```python
from build123d import *

# Parameters (mm, degrees)
F1_DEPTH = 6.35
F2_R     = 2.53999


# Not quite as in the source:
# - a fillet or chamfer is up to 0.001 mm smaller than in the source, because OpenCascade refuses the exact size


with BuildPart() as f1:
    # F0 (on Top) → F1 (new body)
    with BuildSketch(Plane.XY):
        with BuildLine():
            ThreePointArc((6.76275, -11.7134265989), (11.7134265989, -6.76275), (13.5255, 0))
            ThreePointArc((13.5255, 0), (11.7134265989, 6.76275), (6.76275, 11.7134265989))
            ThreePointArc((6.76275, 11.7134265989), (3.5006569945, 13.0646297635), (0, 13.5255))
            Line((0, 13.5255), (0, 10.9855))
            ThreePointArc((0, 10.9855), (7.7679215447, 7.7679215447), (10.9855, 0))
            ThreePointArc((10.9855, 0), (7.7679215447, -7.7679215447), (0, -10.9855))
            Line((0, -10.9855), (0, -13.5255))
            ThreePointArc((0, -13.5255), (3.5006569945, -13.0646297635), (6.76275, -11.7134265989))
        make_face()
        with BuildLine():
            Line((13.5255, -7.8089510659), (13.5255, 0))
            ThreePointArc((13.5255, 0), (11.7134265989, -6.76275), (6.76275, -11.7134265989))
            Line((6.76275, -11.7134265989), (13.5255, -7.8089510659))
        make_face()
        with BuildLine():
            ThreePointArc((6.76275, 11.7134265989), (11.7134265989, 6.76275), (13.5255, 0))
            Line((13.5255, 0), (13.5255, 7.8089510659))
            Line((13.5255, 7.8089510659), (6.76275, 11.7134265989))
        make_face()
        with BuildLine():
            ThreePointArc((0, 13.5255), (3.5006569945, 13.0646297635), (6.76275, 11.7134265989))
            Line((6.76275, 11.7134265989), (0.6545456927, 15.24))
            Line((0.6545456927, 15.24), (0, 14.8620978682))
            Line((0, 14.8620978682), (0, 13.5255))
        make_face()
        Polygon((0.6545456927, 15.24), (6.76275, 11.7134265989), (6.76275, 18.7665734011), align=None)
        with BuildLine():
            Line((0.6545456927, -15.24), (6.76275, -11.7134265989))
            ThreePointArc((6.76275, -11.7134265989), (3.5006569945, -13.0646297635), (0, -13.5255))
            Line((0, -13.5255), (0, -14.8620978682))
            Line((0, -14.8620978682), (0.6545456927, -15.24))
        make_face()
        Polygon((6.76275, -18.7665734011), (6.76275, -11.7134265989), (0.6545456927, -15.24), align=None)
        with BuildLine():
            Line((0, 10.9855), (0, 13.5255))
            ThreePointArc((0, 13.5255), (-3.5006569945, 13.0646297635), (-6.76275, 11.7134265989))
            ThreePointArc((-6.76275, 11.7134265989), (-11.7134265989, 6.76275), (-13.5255, 0))
            ThreePointArc((-13.5255, 0), (-11.7134265989, -6.76275), (-6.76275, -11.7134265989))
            ThreePointArc((-6.76275, -11.7134265989), (-3.5006569945, -13.0646297635), (0, -13.5255))
            Line((0, -13.5255), (0, -10.9855))
            ThreePointArc((0, -10.9855), (-10.9855, 0), (0, 10.9855))
        make_face()
        with BuildLine():
            ThreePointArc((-6.76275, 11.7134265989), (-3.5006569945, 13.0646297635), (0, 13.5255))
            Line((0, 13.5255), (0, 14.8620978682))
            Line((0, 14.8620978682), (-0.6545456927, 15.24))
            Line((-0.6545456927, 15.24), (-6.76275, 11.7134265989))
        make_face()
        with BuildLine():
            Line((0, 15.6179021318), (0.6545456927, 15.24))
            Line((0.6545456927, 15.24), (6.76275, 18.7665734011))
            ThreePointArc((6.76275, 18.7665734011), (3.5006569945, 17.4153702365), (0, 16.9545))
            Line((0, 16.9545), (0, 15.6179021318))
        make_face()
        with BuildLine():
            ThreePointArc((0, 16.9545), (3.5006569945, 17.4153702365), (6.76275, 18.7665734011))
            ThreePointArc((6.76275, 18.7665734011), (11.7134265989, 23.71725), (13.5255, 30.48))
            ThreePointArc((13.5255, 30.48), (11.7134266013, 37.2427499958), (6.7627500083, 42.1934265941))
            ThreePointArc((6.7627500083, 42.1934265941), (-1.056e-07, 44.0055), (-6.7627501912, 42.1934264885))
            ThreePointArc((-6.7627501912, 42.1934264885), (-11.7134266541, 37.2427499044), (-13.5255, 30.48))
            ThreePointArc((-13.5255, 30.48), (-11.7134265989, 23.71725), (-6.76275, 18.7665734011))
            ThreePointArc((-6.76275, 18.7665734011), (-3.5006569945, 17.4153702365), (0, 16.9545))
        make_face()
        with BuildLine():
            ThreePointArc((10.9855, 30.48), (7.7679215447, 22.7120784553), (0, 19.4945))
            ThreePointArc((0, 19.4945), (-7.7679215447, 38.2479215447), (10.9855, 30.48))
        make_face(mode=Mode.SUBTRACT)
        with BuildLine():
            ThreePointArc((13.5255, 30.48), (11.7134265989, 23.71725), (6.76275, 18.7665734011))
            Line((6.76275, 18.7665734011), (13.5255, 22.6710489341))
            Line((13.5255, 22.6710489341), (13.5255, 30.48))
        make_face()
        with BuildLine():
            Line((0, -14.8620978682), (0, -13.5255))
            ThreePointArc((0, -13.5255), (-3.5006569945, -13.0646297635), (-6.76275, -11.7134265989))
            Line((-6.76275, -11.7134265989), (-0.6545456927, -15.24))
            Line((-0.6545456927, -15.24), (0, -14.8620978682))
        make_face()
        with BuildLine():
            Line((6.76275, -18.7665734011), (0.6545456927, -15.24))
            Line((0.6545456927, -15.24), (0, -15.6179021318))
            Line((0, -15.6179021318), (0, -16.9545))
            ThreePointArc((0, -16.9545), (3.5006569945, -17.4153702365), (6.76275, -18.7665734011))
        make_face()
        with BuildLine():
            Line((13.5255, -22.6710489341), (6.76275, -18.7665734011))
            ThreePointArc((6.76275, -18.7665734011), (11.7134265989, -23.71725), (13.5255, -30.48))
            Line((13.5255, -30.48), (13.5255, -22.6710489341))
        make_face()
        with BuildLine():
            ThreePointArc((13.5255, -30.48), (11.7134265989, -23.71725), (6.76275, -18.7665734011))
            ThreePointArc((6.76275, -18.7665734011), (3.5006569945, -17.4153702365), (0, -16.9545))
            ThreePointArc((0, -16.9545), (-3.5006569945, -17.4153702365), (-6.76275, -18.7665734011))
            ThreePointArc((-6.76275, -18.7665734011), (-11.7134265989, -23.71725), (-13.5255, -30.48))
            ThreePointArc((-13.5255, -30.48), (-11.7134266419, -37.2427499255), (-6.762750149, -42.1934265129))
            ThreePointArc((-6.762750149, -42.1934265129), (-1.97e-07, -44.0055), (6.7627498078, -42.1934267099))
            ThreePointArc((6.7627498078, -42.1934267099), (11.7134265434, -37.2427500961), (13.5255, -30.48))
        make_face()
        with BuildLine():
            ThreePointArc((10.9855, -30.48), (-7.7679215447, -38.2479215447), (0, -19.4945))
            ThreePointArc((0, -19.4945), (7.7679215447, -22.7120784553), (10.9855, -30.48))
        make_face(mode=Mode.SUBTRACT)
        with BuildLine():
            ThreePointArc((-13.5255, 0), (-11.7134265989, 6.76275), (-6.76275, 11.7134265989))
            Line((-6.76275, 11.7134265989), (-13.5255, 7.8089510659))
            Line((-13.5255, 7.8089510659), (-13.5255, 0))
        make_face()
        Polygon((-6.76275, 18.7665734011), (-6.76275, 11.7134265989), (-0.6545456927, 15.24), align=None)
        with BuildLine():
            Line((-0.6545456927, 15.24), (0, 15.6179021318))
            Line((0, 15.6179021318), (0, 16.9545))
            ThreePointArc((0, 16.9545), (-3.5006569945, 17.4153702365), (-6.76275, 18.7665734011))
            Line((-6.76275, 18.7665734011), (-0.6545456927, 15.24))
        make_face()
        with BuildLine():
            ThreePointArc((6.7627500083, 42.1934265941), (11.7134266013, 37.2427499958), (13.5255, 30.48))
            Line((13.5255, 30.48), (13.5255, 38.2889510659))
            Line((13.5255, 38.2889510659), (6.7627500083, 42.1934265941))
        make_face()
        with BuildLine():
            Line((-13.5255, -7.8089510659), (-6.76275, -11.7134265989))
            ThreePointArc((-6.76275, -11.7134265989), (-11.7134265989, -6.76275), (-13.5255, 0))
            Line((-13.5255, 0), (-13.5255, -7.8089510659))
        make_face()
        Polygon((-0.6545456927, -15.24), (-6.76275, -11.7134265989), (-6.76275, -18.7665734011), align=None)
        with BuildLine():
            Line((0, -16.9545), (0, -15.6179021318))
            Line((0, -15.6179021318), (-0.6545456927, -15.24))
            Line((-0.6545456927, -15.24), (-6.76275, -18.7665734011))
            ThreePointArc((-6.76275, -18.7665734011), (-3.5006569945, -17.4153702365), (0, -16.9545))
        make_face()
        with BuildLine():
            Line((13.5255, -38.2889510659), (13.5255, -30.48))
            ThreePointArc((13.5255, -30.48), (11.7134265434, -37.2427500961), (6.7627498078, -42.1934267099))
            Line((6.7627498078, -42.1934267099), (13.5255, -38.2889510659))
        make_face()
        with BuildLine():
            Line((-13.5255, 22.6710489341), (-6.76275, 18.7665734011))
            ThreePointArc((-6.76275, 18.7665734011), (-11.7134265989, 23.71725), (-13.5255, 30.48))
            Line((-13.5255, 30.48), (-13.5255, 22.6710489341))
        make_face()
        with BuildLine():
            ThreePointArc((-6.7627501912, 42.1934264885), (-1.056e-07, 44.0055), (6.7627500083, 42.1934265941))
            Line((6.7627500083, 42.1934265941), (0, 46.0979021318))
            Line((0, 46.0979021318), (-6.7627501912, 42.1934264885))
        make_face()
        with BuildLine():
            ThreePointArc((-13.5255, -30.48), (-11.7134265989, -23.71725), (-6.76275, -18.7665734011))
            Line((-6.76275, -18.7665734011), (-13.5255, -22.6710489341))
            Line((-13.5255, -22.6710489341), (-13.5255, -30.48))
        make_face()
        with BuildLine():
            Line((0, -46.0979021318), (6.7627498078, -42.1934267099))
            ThreePointArc((6.7627498078, -42.1934267099), (-1.97e-07, -44.0055), (-6.762750149, -42.1934265129))
            Line((-6.762750149, -42.1934265129), (0, -46.0979021318))
        make_face()
        with BuildLine():
            Line((-13.5255, 38.2889510659), (-13.5255, 30.48))
            ThreePointArc((-13.5255, 30.48), (-11.7134266541, 37.2427499044), (-6.7627501912, 42.1934264885))
            Line((-6.7627501912, 42.1934264885), (-13.5255, 38.2889510659))
        make_face()
        with BuildLine():
            ThreePointArc((-6.762750149, -42.1934265129), (-11.7134266419, -37.2427499255), (-13.5255, -30.48))
            Line((-13.5255, -30.48), (-13.5255, -38.2889510659))
            Line((-13.5255, -38.2889510659), (-6.762750149, -42.1934265129))
        make_face()
    extrude(amount=F1_DEPTH)

    # F2 (radius 2.54 in the source; OpenCascade refuses exactly that, so slightly less here)
    f2_edges = [f1.edges().sort_by_distance(p)[0] for p in [
        (-6.76275, -42.193427, 6.35),
        (6.76275, -42.193427, 6.35),
        (13.5255, -30.48, 6.35),
        (-13.5255, -30.48, 6.35),
        (-10.144125, -20.718811, 6.35),
        (-6.76275, -15.24, 6.35),
        (10.144125, -20.718811, 6.35),
        (6.76275, -15.24, 6.35),
        (-10.144125, -9.761189, 6.35),
        (-13.5255, 0, 6.35),
        (-10.144125, 9.761189, 6.35),
        (-6.76275, 15.24, 6.35),
        (-10.144125, 20.718811, 6.35),
        (-13.5255, 30.48, 6.35),
        (-6.76275, 42.193427, 6.35),
        (6.76275, 42.193427, 6.35),
        (13.5255, 30.48, 6.35),
        (6.76275, 15.24, 6.35),
        (10.144125, 20.718811, 6.35),
        (10.144125, 9.761189, 6.35),
        (10.144125, -9.761189, 6.35),
        (13.5255, 0, 6.35),
        (-13.5255, -30.48, 0),
        (-6.76275, -42.193427, 0),
        (6.76275, -42.193427, 0),
        (13.5255, -30.48, 0),
        (10.144125, -20.718811, 0),
        (6.76275, -15.24, 0),
        (-10.144125, -20.718811, 0),
        (-6.76275, -15.24, 0),
        (-13.5255, 0, 0),
        (-10.144125, 9.761189, 0),
        (-6.76275, 15.24, 0),
        (-13.5255, 30.48, 0),
        (-6.76275, 42.193427, 0),
        (6.76275, 42.193427, 0),
        (13.5255, 30.48, 0),
        (10.144125, 20.718811, 0),
        (6.76275, 15.24, 0),
        (10.144125, 9.761189, 0),
        (10.144125, -9.761189, 0),
        (13.5255, 0, 0),
        (-10.144125, 20.718811, 0),
    ]]
    fillet(f2_edges, radius=F2_R)


solid = f1.part
```
For this review, take the finished solid that the model builds, in its own axes (mm). A direction names the side the tool comes from. Give positions to 0.01 mm unless a question says otherwise; leave off trailing zeros. Write each loop counter-clockwise with the first axis right and the second up, starting at its lowest first coordinate (ties: lowest second). Pieces come first, ordered by that corner, then holes. Notation, with made-up numbers: M -24.75,60.5 L 12.25,60.5 A23 ccw 12.25,92.5 Z; hole C 84.5,28.25 d2. An arc over 180 degrees is marked long. Answer as a JSON object with one key per item and string values. Group by question number.
Item 1: Consider section B-B on y = -27. Write out the cut boundary in (x, z).
Item 2: Consider section A-A on y = 34. Write out the cut boundary in (x, z), plus the area to 3 significant figures.
Item 3: Draft analysis for pull direction Y (two halves, no side actions). For faces 5 (the cylindrical face through (-9.203, -21.012, 0.764)), 6 (the cylindrical face through (-12.8, 30.37, 5.59)), state which applies: +Y half, -Y half, draft (parallel to the pull), parting line (faces both ways), or undercut.
Item 4: For pin 1 Ø6 at (x, y) = (-7.5, -24) entering from -Z; pin 2 Ø1 at (y, z) = (-14.5, 3) entering from -X; pin 3 Ø1.4 at (y, z) = (15, 3) entering from +X, all flat-tipped, find the tip position at first contact; note any pin that passes through.
Item 5: For probe 1 along X at (y, z) = (30.48, 3.5); probe 2 along Y at (x, z) = (-5.75, 3.5); probe 3 along Y at (x, z) = (7.5, 1.5), list the stretches that pass through material, from the lowest coordinate up. Write a range as [from, to].
Item 6: Tool access review of faces 1 (the cylindrical face through (6.038, -15.17, 5.586)), 2 (the cylindrical face through (9.09, 9.53, 0.76)), 3 (the cylindrical face through (-6.038, 15.17, 5.586)), 4 (the cylindrical face through (-6.038, 15.17, 0.764)): name each direction out of +Z, -Z, +X, -X, +Y, -Y from which nothing blocks a thin tool from reaching the whole face with its end or side.
Item 7: Consider section C-C on z = 5. Count the separate pieces of the cut face and the enclosed holes in it, plus the area to 3 significant figures.
Check result:
{
 "1": {"outline": "M -13.53,2.54 A2.54 ccw -10.99,0 L -10.42,0 L -10.42,6.35 L -10.99,6.35 A2.54 ccw -13.53,3.81 Z; M 10.42,0 L 10.99,0 A2.54 ccw 13.53,2.54 L 13.53,3.81 A2.54 ccw 10.99,6.35 L 10.42,6.35 Z"},
 "2": {"outline": "M -13.53,2.54 A2.54 ccw -10.99,0 L -10.41,0 L -10.41,6.35 L -10.99,6.35 A2.54 ccw -13.53,3.81 Z; M 10.41,0 L 10.99,0 A2.54 ccw 13.53,2.54 L 13.53,3.81 A2.54 ccw 10.99,6.35 L 10.41,6.35 Z", "area": "34.1 mm^2"},
 "3": {"face 5": "undercut", "face 6": "draft"},
 "4": {"pin 1": "stops at z = 0", "pin 2": "stops at x = -6.76", "pin 3": "stops at x = 6.76"},
 "5": {"probe 1": "x = [-13.53, -10.99], [10.99, 13.53]", "probe 2": "y = [-42.78, -39.84], [-21.12, -9.36], [9.36, 21.12], [39.84, 42.78]", "probe 3": "y = [-41.51, -38.51], [-22.45, -19.45], [-11.03, -8.03], [8.03, 11.03], [19.45, 22.45], [38.51, 41.51]"},
 "6": {"face 1": "+Z, +X", "face 2": "-Z, +X", "face 3": "+Z, -X", "face 4": "-Z, -X"},
 "7": {"separate pieces": "1", "enclosed holes": "5", "area": "775 mm^2"}
}
